For this review, use the dimensioned drawing (mm, ordinates from the lowest corner) and the shaded views. A direction names the side the tool comes from. Coordinates: 2 decimals unless noted, no trailing zeros. Loops run counter-clockwise (first coordinate to the right, second up) from the corner with the lowest first, then second, coordinate; pieces in that order, holes last.
1. Take a section at C-C, the plane x = 44. State the section outline as (y, z) points, then the cut area to 3 significant figures.
2. Clearance check with flat-ended pins moving along their axes: P1, Ø5, axis at x = 91, z = 11, coming from the -Y side; P2, Ø1, axis at y = 11.5, z = 55, coming from the +X side. State where each tip first meets the part, or that it passes through.
3. To check wall thickness, follow probe 1 along Y at (x, z) = (8, 69); probe 2 along X at (y, z) = (3, 44.5) (1 decimal). State the ranges of each line that lie inside material, in increasing order.
4. Mouldability with a two-part tool opening along X and no side actions: class the marked faces 3, 4 and 5 as pulls with the +X half, pulls with the -X half, needs draft (parallel to the pull), parting line crosses it, or undercut.
5. Take a section at A-A, the plane y = 9. State the section outline as (x, z) points (1 decimal).
6. Take a section at B-B, the plane z = 38.1. State the section outline as (x, y) points.
7. Take a section at D-D, the plane x = 79. State the section outline as (y, z) points, then the cut area to 3 significant figures.
8. Machinability: for the marked faces 1 and 2, which of the approach directions +Z, -Z, +X, -X, +Y, -Y give a long, thin tool a straight path to every point of the face, cutting with its end or side? Answer none if there is none.
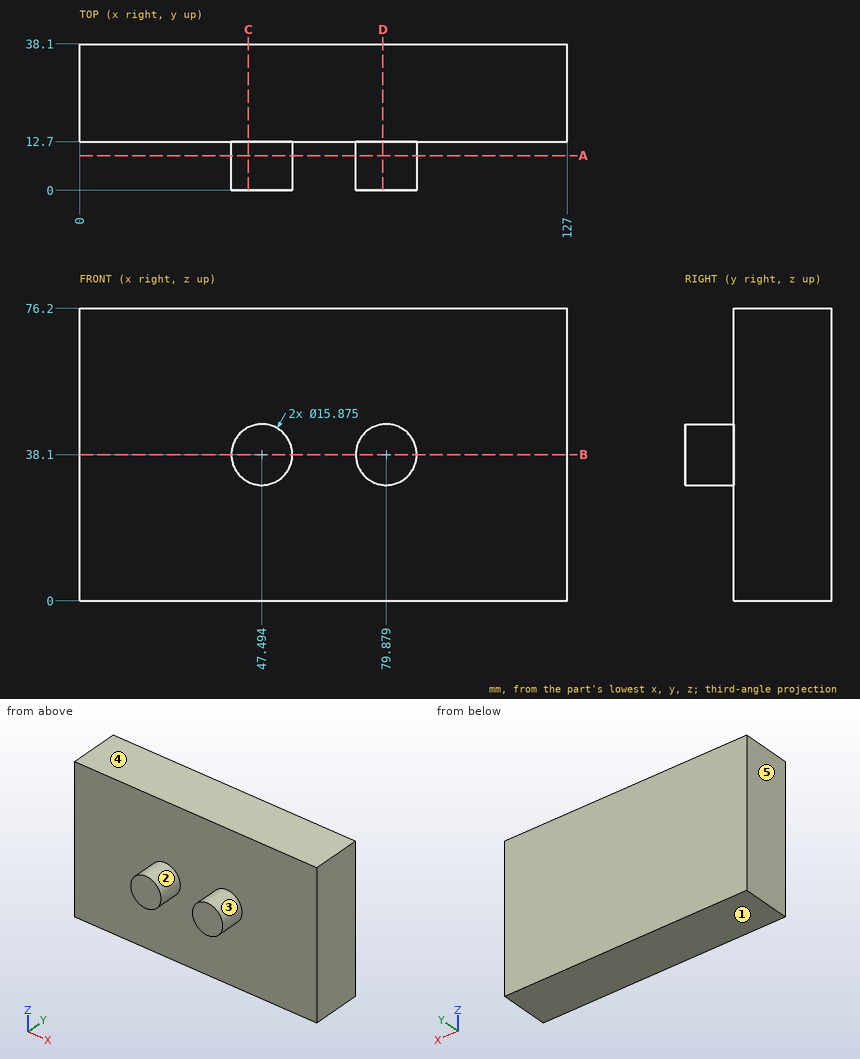
Results list:
1. outline: (0, 30.97) - (12.7, 30.97) - (12.7, 0) - (38.1, 0) - (38.1, 76.2) - (12.7, 76.2) - (12.7, 45.23) - (0, 45.23) - close
1. area: 2,120 mm2
2. P1: stops at y = 12.7
2. P2: passes through
3. probe 1: y = 12.7 to 38.1
3. probe 2: x = 42.8 to 52.2, 75.2 to 84.6
4. face 3: undercut
4. face 4: needs draft
4. face 5: pulls with the -X half
5. outline: circle Ø15.9 at (47.5, 38.1); circle Ø15.9 at (79.9, 38.1)
6. outline: (0, 12.7) - (39.56, 12.7) - (39.56, 0) - (55.43, 0) - (55.43, 12.7) - (71.94, 12.7) - (71.94, 0) - (87.82, 0) - (87.82, 12.7) - (127, 12.7) - (127, 38.1) - (0, 38.1) - close
7. outline: (0, 30.21) - (12.7, 30.21) - (12.7, 0) - (38.1, 0) - (38.1, 76.2) - (12.7, 76.2) - (12.7, 45.99) - (0, 45.99) - close
7. area: 2,140 mm2
8. face 1: -Z, +X, -X, +Y, -Y
8. face 2: -Y
